```python
from build123d import *

# Parameters (mm, degrees)
BOSS_EXTRUDE1_DEPTH                = 38
CUT_EXTRUDE1_DEPTH                 = 30
CUT_EXTRUDE2_DEPTH                 = 5
SKETCH4_W                          = 19.9
SKETCH4_H                          = 38
BOSS_EXTRUDE2_DEPTH                = 7.5
SKETCH5_W                          = 19.9
SKETCH5_H                          = 38
BOSS_EXTRUDE3_DEPTH                = 7.5
CUT_EXTRUDE3_DEPTH                 = 30
CUT_EXTRUDE4_DEPTH                 = 30
SKETCH8_W                          = 44
SKETCH8_H                          = 165
BOSS_EXTRUDE4_DEPTH                = 2
SKETCH9_W                          = 18
SKETCH9_H                          = 3
F_4_0_4_DIAMETER_HOLE1_D           = 4
F_4_0_4_DIAMETER_HOLE1_DEPTH       = 38
F_4_0_4_DIAMETER_HOLE2_D           = 4
F_4_0_4_DIAMETER_HOLE2_DEPTH       = 38
F_5_0_5_DIAMETER_HOLE1_D           = 5
F_5_0_5_DIAMETER_HOLE1_DEPTH       = 8
M24_CLEARANCE_HOLE1_D              = 28
F_10_0_10_DIAMETER_HOLE1_D         = 10
F_10_0_10_DIAMETER_HOLE1_DEPTH     = 38
F_5_0_5_DIAMETER_HOLE2_D           = 5
F_5_0_5_DIAMETER_HOLE2_DEPTH       = 5
F_5_0_5_DIAMETER_HOLE2_CSINK_D     = 10.000000842
F_5_0_5_DIAMETER_HOLE2_CSINK_ANGLE = 90.00001
F_5_0_5_DIAMETER_HOLE3_D           = 5
F_5_0_5_DIAMETER_HOLE3_DEPTH       = 6
F_5_0_5_DIAMETER_HOLE4_D           = 5
F_5_0_5_DIAMETER_HOLE4_DEPTH       = 20
F_5_0_5_DIAMETER_HOLE5_D           = 5
F_5_0_5_DIAMETER_HOLE5_DEPTH       = 35
F_5_0_5_DIAMETER_HOLE6_D           = 5
F_5_0_5_DIAMETER_HOLE6_DEPTH       = 30
CHAMFER1_SIZE2                     = 2.499999787
CHAMFER1_SIZE                      = 2.50000021
CHAMFER2_SIZE                      = 1
FILLET1_R                          = 8
FILLET2_R                          = 12
FILLET3_R                          = 15
FILLET4_R                          = 20
SKETCH32_R                         = 14
CUT_EXTRUDE5_DEPTH                 = 6


with BuildPart() as part:
    # Sketch1 → Boss-Extrude1 (new body)
    with BuildSketch(Plane.XY.offset(38)):
        with BuildLine():
            Line((70, 36), (-70, 36))
            Line((-70, 36), (-70, -179.1))
            ThreePointArc((-70, -179.1), (0, -249.1), (70, -179.1))
            Line((70, -179.1), (70, 36))
        make_face()
    extrude(amount=-BOSS_EXTRUDE1_DEPTH)

    # Sketch2 → Cut-Extrude1 (cut)
    with BuildSketch(Plane.XY.offset(38)):
        with BuildLine():
            Line((-38.1, 36), (-38.1, 30))
            Line((-38.1, 30), (-65, 30))
            Line((-65, 30), (-65, -34.583920217))
            ThreePointArc((-65, -34.583920217), (-58.354610186, -38.467864707), (-61, -45.696152423))
            ThreePointArc((-61, -45.696152423), (-63.92820323, -48.624355653), (-65, -52.624355653))
            Line((-65, -52.624355653), (-65, -124.083920217))
            ThreePointArc((-65, -124.083920217), (-58.211536441, -128.420857946), (-61.857142857, -135.604298642))
            ThreePointArc((-61.857142857, -135.604298642), (-65.590035768, -138.541123155), (-67, -143.076696831))
            Line((-67, -143.076696831), (-67, -177.5))
            ThreePointArc((-67, -177.5), (0, -244.5), (67, -177.5))
            Line((67, -177.5), (67, -143.076696831))
            ThreePointArc((67, -143.076696831), (65.590035768, -138.541123155), (61.857142857, -135.604298642))
            ThreePointArc((61.857142857, -135.604298642), (58.211536441, -128.420857946), (65, -124.083920217))
            Line((65, -124.083920217), (65, -52.624355653))
            ThreePointArc((65, -52.624355653), (63.92820323, -48.624355653), (61, -45.696152423))
            ThreePointArc((61, -45.696152423), (58.354610186, -38.467864707), (65, -34.583920217))
            Line((65, -34.583920217), (65, 30))
            Line((65, 30), (38.1, 30))
            Line((38.1, 30), (38.1, 36))
            Line((38.1, 36), (-38.1, 36))
        make_face()
    extrude(amount=-CUT_EXTRUDE1_DEPTH, mode=Mode.SUBTRACT)

    # Sketch3 → Cut-Extrude2 (cut)
    with BuildSketch(Plane.XY.offset(8)):
        with BuildLine():
            Line((56.928932188, -44.5), (-56.928932188, -44.5))
            ThreePointArc((-56.928932188, -44.5), (-58.97017364, -44.783121635), (-60.857303195, -45.611111111))
            ThreePointArc((-60.857303195, -45.611111111), (-60.928357277, -45.654125627), (-61, -45.696152423))
            ThreePointArc((-61, -45.696152423), (-63.92820323, -48.624355653), (-65, -52.624355653))
            Line((-65, -52.624355653), (-65, -124.083920217))
            ThreePointArc((-65, -124.083920217), (-58.211536441, -128.420857946), (-61.857142857, -135.604298642))
            ThreePointArc((-61.857142857, -135.604298642), (-65.590035768, -138.541123155), (-67, -143.076696831))
            Line((-67, -143.076696831), (-67, -177.5))
            ThreePointArc((-67, -177.5), (0, -244.5), (67, -177.5))
            Line((67, -177.5), (67, -143.076696831))
            ThreePointArc((67, -143.076696831), (65.590035768, -138.541123155), (61.857142857, -135.604298642))
            ThreePointArc((61.857142857, -135.604298642), (58.211536441, -128.420857946), (65, -124.083920217))
            Line((65, -124.083920217), (65, -52.624355653))
            ThreePointArc((65, -52.624355653), (63.92820323, -48.624355653), (61, -45.696152423))
            ThreePointArc((61, -45.696152423), (60.928357277, -45.654125627), (60.857303195, -45.611111111))
            ThreePointArc((60.857303195, -45.611111111), (58.97017364, -44.783121635), (56.928932188, -44.5))
        make_face()
    extrude(amount=-CUT_EXTRUDE2_DEPTH, mode=Mode.SUBTRACT)

    # Sketch4 → Boss-Extrude2 (add)
    with BuildSketch(Plane(origin=(0, 36, 0), x_dir=(-1, 0, 0), z_dir=(0, 1, 0))):
        with Locations((-60.05, 19)):
            Rectangle(SKETCH4_W, SKETCH4_H)
    extrude(amount=BOSS_EXTRUDE2_DEPTH)

    # Sketch5 → Boss-Extrude3 (add)
    with BuildSketch(Plane(origin=(0, 36, 0), x_dir=(-1, 0, 0), z_dir=(0, 1, 0))):
        with Locations((60.05, 19)):
            Rectangle(SKETCH5_W, SKETCH5_H)
    extrude(amount=BOSS_EXTRUDE3_DEPTH)

    # Sketch6 → Cut-Extrude3 (cut)
    with BuildSketch(Plane.XY.offset(38)):
        with BuildLine():
            Line((-65, 30), (-62.677124344, 30))
            ThreePointArc((-62.677124344, 30), (-64.198806606, 33.490094453), (-65, 29.767949192))
            Line((-65, 29.767949192), (-65, 30))
        make_face()
    extrude(amount=-CUT_EXTRUDE3_DEPTH, mode=Mode.SUBTRACT)

    # Sketch7 → Cut-Extrude4 (cut)
    with BuildSketch(Plane.XY.offset(38)):
        with BuildLine():
            Line((65, 30), (65, 29.767949192))
            ThreePointArc((65, 29.767949192), (64.198806606, 33.490094453), (62.677124344, 30))
            Line((62.677124344, 30), (65, 30))
        make_face()
    extrude(amount=-CUT_EXTRUDE4_DEPTH, mode=Mode.SUBTRACT)

    # Sketch8 → Boss-Extrude4 (add)
    with BuildSketch(Plane.XY.offset(3)):
        with Locations((0, -127)):
            Rectangle(SKETCH8_W, SKETCH8_H)
    extrude(amount=BOSS_EXTRUDE4_DEPTH)

    # Sketch9 → Revolve1 (revolve)
    with BuildSketch(Plane.XZ):
        with Locations((9, 9.5)):
            Rectangle(SKETCH9_W, SKETCH9_H)
    revolve(axis=Axis((0, 0, 11), (0, 0, -1)))

    # Sketch10 → Revolve2 (revolve)
    with BuildSketch(Plane.XZ.offset(179.1)):
        Polygon((11.98, 30), (0, 30), (0, 5), (19, 5), (19, 6), (12.48, 6), (12.48, 19), (11.98, 19.575184204), align=None)
    revolve(axis=Axis((0, -179.1, 30), (0, 0, -1)))

    # Sketch11 → Cut-Revolve1 (revolve, cut)
    with BuildSketch(Plane.XZ):
        Polygon((14, 11), (0, 11), (0, 0), (14, 0), (14, 8), (14.75, 8), (14.75, 9.3), (14, 9.3), align=None)
    revolve(axis=Axis((0, 0, 11), (0, 0, -1)), mode=Mode.SUBTRACT)

    # 4.0 _4_ Diameter Hole1
    with Locations(Plane(origin=(0, 0, 0), x_dir=(-1, 0, 0), z_dir=(0, 0, -1))):
        with Locations((-16.5, -177.5), (16.5, -177.5)):
            Hole(F_4_0_4_DIAMETER_HOLE1_D / 2, depth=F_4_0_4_DIAMETER_HOLE1_DEPTH)

    # 4.0 _4_ Diameter Hole2
    with Locations(Plane(origin=(0, 0, 0), x_dir=(-1, 0, 0), z_dir=(0, 0, -1))):
        with Locations((0, -40.5)):
            Hole(F_4_0_4_DIAMETER_HOLE2_D / 2, depth=F_4_0_4_DIAMETER_HOLE2_DEPTH)

    # 5.0 _5_ Diameter Hole1
    with Locations(Plane.XY.offset(8)):
        with Locations((14, -26), (-14, -26), (0, 27)):
            Hole(F_5_0_5_DIAMETER_HOLE1_D / 2, depth=F_5_0_5_DIAMETER_HOLE1_DEPTH)

    # M24 Clearance Hole1 (through all)
    with Locations(Plane.XY.offset(5)):
        with Locations((0, -85)):
            Hole(M24_CLEARANCE_HOLE1_D / 2)

    # 10.0 _10_ Diameter Hole1
    with Locations(Plane(origin=(0, 0, 0), x_dir=(-1, 0, 0), z_dir=(0, 0, -1))):
        with Locations((0, -177.5)):
            Hole(F_10_0_10_DIAMETER_HOLE1_D / 2, depth=F_10_0_10_DIAMETER_HOLE1_DEPTH)

    # 5.0 _5_ Diameter Hole2
    with Locations(Plane.XY.offset(5)):
        with Locations((14, -201), (-14, -201), (-14, -152), (14, -152), (-14, -110), (14, -110), (-14, -58), (14, -58)):
            CounterSinkHole(F_5_0_5_DIAMETER_HOLE2_D / 2, F_5_0_5_DIAMETER_HOLE2_CSINK_D / 2, depth=F_5_0_5_DIAMETER_HOLE2_DEPTH, counter_sink_angle=F_5_0_5_DIAMETER_HOLE2_CSINK_ANGLE)

    # 5.0 _5_ Diameter Hole3
    with Locations(Plane(origin=(0, 36, 0), x_dir=(1, 0, 0), z_dir=(0, 1, 0))):
        with Locations((44, -14), (44, -32), (-44, -32), (-44, -14)):
            Hole(F_5_0_5_DIAMETER_HOLE3_D / 2, depth=F_5_0_5_DIAMETER_HOLE3_DEPTH)

    # 5.0 _5_ Diameter Hole4
    with Locations(Plane(origin=(0, 36, 0), x_dir=(1, 0, 0), z_dir=(0, 1, 0))):
        with Locations((28, -4), (-28, -4)):
            Hole(F_5_0_5_DIAMETER_HOLE4_D / 2, depth=F_5_0_5_DIAMETER_HOLE4_DEPTH)

    # 5.0 _5_ Diameter Hole5
    with Locations(Plane.XY.offset(38)):
        with Locations((64, -130), (-64, -130)):
            Hole(F_5_0_5_DIAMETER_HOLE5_D / 2, depth=F_5_0_5_DIAMETER_HOLE5_DEPTH)

    # 5.0 _5_ Diameter Hole6
    with Locations(Plane.XY.offset(38)):
        with Locations((-56, 35.5), (56, 35.5), (64, -40.5), (-64, -40.5)):
            Hole(F_5_0_5_DIAMETER_HOLE6_D / 2, depth=F_5_0_5_DIAMETER_HOLE6_DEPTH)

    # Chamfer1
    chamfer1_edges = [part.edges().sort_by_distance(p)[0] for p in [
        (2.5, 27, 8),
        (-11.5, -26, 8),
        (16.5, -26, 8),
    ]]
    chamfer(chamfer1_edges, length=CHAMFER1_SIZE, length2=CHAMFER1_SIZE2)

    # Chamfer2
    chamfer2_edges = [part.edges().sort_by_distance(p)[0] for p in [
        (-11.98, -179.1, 30),
    ]]
    chamfer(chamfer2_edges, length=CHAMFER2_SIZE)

    # Fillet1
    fillet1_edges = [part.edges().sort_by_distance(p)[0] for p in [
        (65, -34.583920217, 23),
        (65, -124.083920217, 20.5),
        (-65, -124.083920217, 20.5),
        (-65, -34.583920217, 23),
    ]]
    fillet(fillet1_edges, radius=FILLET1_R)

    # Fillet2
    fillet2_edges = [part.edges().sort_by_distance(p)[0] for p in [
        (-22, -209.5, 4),
        (22, -209.5, 4),
    ]]
    fillet(fillet2_edges, radius=FILLET2_R)

    # Fillet3
    fillet3_edges = [part.edges().sort_by_distance(p)[0] for p in [
        (70, 43.5, 19),
        (-70, 43.5, 19),
    ]]
    fillet(fillet3_edges, radius=FILLET3_R)

    # Fillet4
    fillet4_edges = [part.edges().sort_by_distance(p)[0] for p in [
        (22, -44.5, 4),
        (-22, -44.5, 4),
    ]]
    fillet(fillet4_edges, radius=FILLET4_R)

    # Sketch32 → Cut-Extrude5 (cut, through all)
    with BuildSketch(Plane.XY.offset(5)):
        with Locations((0, -85.75)):
            Circle(SKETCH32_R)
    extrude(amount=-CUT_EXTRUDE5_DEPTH, mode=Mode.SUBTRACT)


solid = part.part
```
Build history of the part. All positions in model axes, mm. A direction names the side the tool comes from. Round coordinates to 2 decimals unless told otherwise and drop trailing zeros. Write each loop counter-clockwise with the first axis right and the second up, starting at its lowest first coordinate (ties: lowest second). Pieces come first, ordered by that corner, then holes.
1) Drill centre lines: probe 1 along X at (y, z) = (-41, 9); probe 2 along Y at (x, z) = (-56.5, 20); probe 3 along Z at (x, y) = (28, 25.75). Where is each one in solid material? Low to high.
2) Pin check, flat tips, straight feed: pin 1 (6 mm diameter, centred on x = 0, y = -177.5, fed in from -Z); pin 2 (8 mm diameter, centred on y = 40.5, z = 14, fed in from +X); pin 3 (24 mm diameter, centred on x = 2, y = -180, fed in from +Z); pin 4 (8 mm diameter, centred on y = 39, z = 12.5, fed in from -X). Stop position of each tip, or through.
3) Band-saw the part on A-A, the plane y = 0. List the corners of the cut face in (x, z), and give its area (3 significant figures).
4) 3-axis set-ups, long thin cutter, end or side, ignore diameter. For faces 3 (the cylindrical face through (15.84, -24.31, 2.71)), 4 (the cylindrical face through (6.709, -189.623, 12.591)): which of +Z, -Z, +X, -X, +Y, -Y reach the whole face in a straight line?
5) Band-saw the part on B-B, the plane y = -220. List the corners of the cut face in (x, z).
6) Mould opens along Y. For faces 1 (the flat face through (-64, -40, 8)), 2 (the flat face through (-9, 11, 11)) say: +Y half, -Y half, draft (parallel to the pull), parting line (faces both ways), or undercut.
Ans:
1. probe 1: x = -70 to -66.45, -61.55 to -58.02, 58.02 to 61.55, 66.45 to 70
1. probe 2: y = -220.42 to -213.51, 30 to 33.05, 37.95 to 43.42
1. probe 3: z = 0 to 1.5, 6.5 to 8
2. pin 1: passes through
2. pin 2: stops at x = 67.69
2. pin 3: stops at z = 30
2. pin 4: stops at x = -68.52
3. outline: (-70, 0) - (-14, 0) - (-14, 8) - (-14.75, 8) - (-14.75, 9.3) - (-14, 9.3) - (-14, 11) - (-18, 11) - (-18, 8) - (-65, 8) - (-65, 38) - (-70, 38) - close; (14, 0) - (70, 0) - (70, 38) - (65, 38) - (65, 8) - (18, 8) - (18, 11) - (14, 11) - (14, 9.3) - (14.75, 9.3) - (14.75, 8) - (14, 8) - close
3. area: 1,220 mm2
4. face 3: +Z, -Z
4. face 4: +Z
5. outline: (-56.81, 0) - (56.81, 0) - (56.81, 38) - (51.8, 38) - (51.8, 3) - (-51.8, 3) - (-51.8, 38) - (-56.81, 38) - close
6. face 1: undercut
6. face 2: draft
